Design review of the part shown in the three views and the two pictorial views. Dimensions are in mm from the part's minimum x, y and z. A direction names the side the tool comes from. Coordinates: 2 decimals unless noted, no trailing zeros. Loops run counter-clockwise (first coordinate to the right, second up) from the corner with the lowest first, then second, coordinate; pieces in that order, holes last. Notation, with made-up numbers: (2, -0.5) -> (10, -0.5) arc R6 ccw to (10, 8.5) -> close; hole circle Ø3 at (80, 43.5). An arc over 180 degrees is marked (long way). Answer in a Markdown table with one row per item.
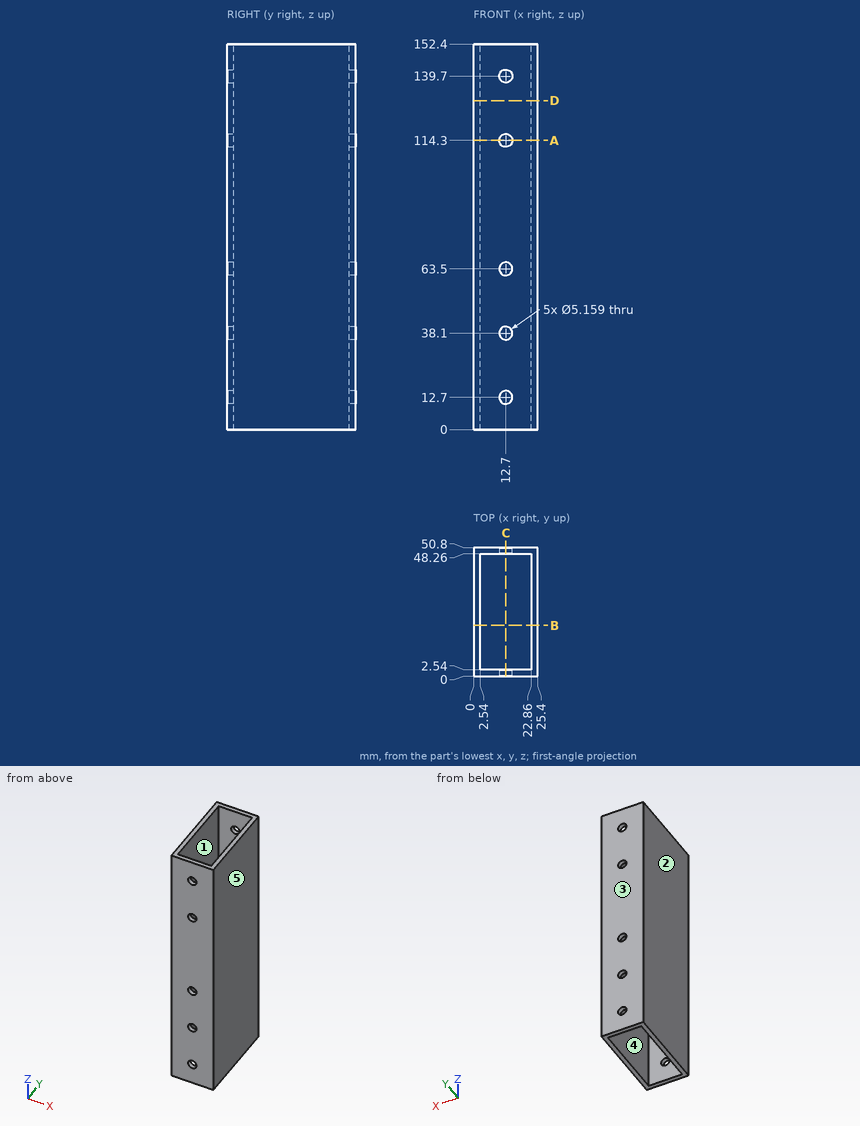
Item 1: Take a section at B-B, the plane y = 20. State the section outline as (x, z) points.
Worked answers:
| item | result |
|---|---|
| outline | (0, 0) -> (2.54, 0) -> (2.54, 152.4) -> (0, 152.4) -> close; (22.86, 0) -> (25.4, 0) -> (25.4, 152.4) -> (22.86, 152.4) -> close |
Item 2: Take a section at A-A, the plane z = 114.3. State the section outline as (x, y) points.
Worked answers:
| item | result |
|---|---|
| outline | (0, 0) -> (10.12, 0) -> (10.12, 2.54) -> (2.54, 2.54) -> (2.54, 48.26) -> (10.12, 48.26) -> (10.12, 50.8) -> (0, 50.8) -> close; (15.28, 0) -> (25.4, 0) -> (25.4, 50.8) -> (15.28, 50.8) -> (15.28, 48.26) -> (22.86, 48.26) -> (22.86, 2.54) -> (15.28, 2.54) -> close |
Item 3: For the marked faces 4 and 5, list the 3-axis set-ups (+Z, -Z, +X, -X, +Y, -Y) from which the entire face can be reached by the end or side of a thin tool; tool diameter is ignored.
Worked answers:
| item | result |
|---|---|
| face 4 | +Z, -Z |
| face 5 | +Z, -Z, +X, +Y, -Y |
Item 4: Insertion check: pin 1 (3 mm diameter, centred on x = 12.7, z = 63.5, fed in from -Y); pin 2 (8.5 mm diameter, centred on x = 12.7, z = 12.7, fed in from -Y). Each pin has a flat end and moves straight along its axis. Give the tip position at first contact, or say it passes through.
Worked answers:
| item | result |
|---|---|
| pin 1 | through |
| pin 2 | y = 0 |
Item 5: Take a section at C-C, the plane x = 12.7. Count the separate pieces of the cut face and the enclosed holes in it.
Worked answers:
| item | result |
|---|---|
| separate pieces | 12 |
| enclosed holes | 0 |
Item 6: Take a section at D-D, the plane z = 130. State the section outline as (x, y) points.
Worked answers:
| item | result |
|---|---|
| outline | (0, 0) -> (25.4, 0) -> (25.4, 50.8) -> (0, 50.8) -> close; hole (2.54, 2.54) -> (22.86, 2.54) -> (22.86, 48.26) -> (2.54, 48.26) -> close |
Item 7: For L1, parallel to Z at x = 12.7, y = 1.15; L2, parallel to X at y = 33, z = 110; L3, parallel to Y at x = 15.5, z = 42.5, list the stretches that pass through material, from the lowest coordinate up.
Worked answers:
| item | result |
|---|---|
| L1 | 0 to 10.12, 15.28 to 35.52, 40.68 to 60.92, 66.08 to 111.72, 116.88 to 137.12, 142.28 to 152.4 |
| L2 | 0 to 2.54, 22.86 to 25.4 |
| L3 | 0 to 2.54, 48.26 to 50.8 |
Item 8: The part is to be moulded in two halves that separate along Y. For the marked faces 1, 2 and 3, say which applies: +Y half, -Y half, draft (parallel to the pull), parting line (faces both ways), or undercut.
Worked answers:
| item | result |
|---|---|
| face 1 | undercut |
| face 2 | draft |
| face 3 | +Y half |
